Verification items for the finished model (mm, model axes). Give positions to 0.01 mm unless a question says otherwise; leave off trailing zeros. Write each loop counter-clockwise with the first axis right and the second up, starting at its lowest first coordinate (ties: lowest second). Pieces come first, ordered by that corner, then holes. Notation, with made-up numbers: (76, 37) -> (103, 37) arc R27 ccw to (103, 67) -> close; hole circle Ø9 at (66, 43). An arc over 180 degrees is marked (long way). Answer as CSV lines item,"result". Start each with the question number.
1) Material ranges on L1, parallel to X at y = 19, z = 0.5; L2, parallel to Z at x = 0, y = -43, recorded low to high.
2) Sectioned sample at A-A on z = 0. Record the cut outline in (x, y), and give its area (3 significant figures).
3) Sectioned sample at B-B on z = -15. Record the cut outline in (x, y), and give its area (3 significant figures).
4) Gauge pin test, flat ends, axial feed: pin 1 Ø10 at (x, y) = (8, -25) entering from -Z; pin 2 Ø12 at (x, y) = (15.5, -35) entering from +Z; pin 3 Ø10.5 at (x, z) = (1, -5) entering from +Y; pin 4 Ø1.5 at (y, z) = (21.5, -7) entering from -X. Record the tip position at first contact, or that the pin passes through.
5) Sectioned sample at C-C on y = -7. Record the cut outline in (x, z) (1 decimal), and give its area (3 significant figures).
6) Sectioned sample at D-D on x = 16.5. Record the cut outline in (y, z).
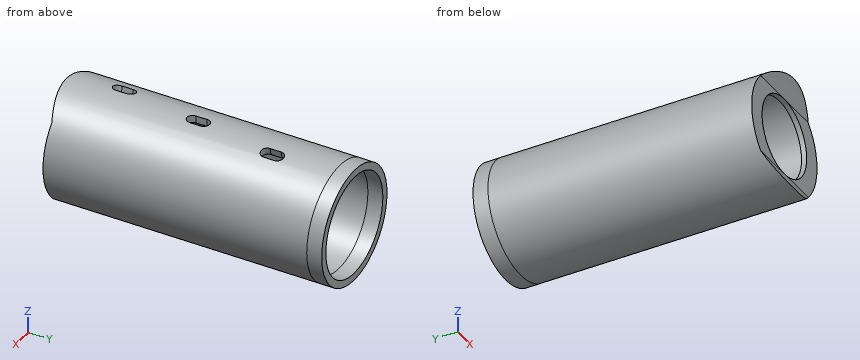
```python
from build123d import *

# Parameters (mm, degrees)
F0_R          = 20.0025
F0_R_2        = 17.4625
F1_DEPTH      = 47.5
F2_R          = 20.0025
F2_R_2        = 13.6525
F3_DEPTH      = 5.08
F5_DEPTH      = 20.0035
F5_DEPTH_BACK = 20.0035
F7_DEPTH      = 20.0035001
F11_DEPTH     = 23.7251510989
F14_DEPTH     = 23.7251510989
F15_R         = 20.0025
F15_R_2       = 17.4625
F16_DEPTH     = 5.207


with BuildPart() as f1:
    # F0 (on Front) → F1 (new body, symmetric)
    with BuildSketch(Plane.XZ):
        Circle(F0_R)
        Circle(F0_R_2, mode=Mode.SUBTRACT)
    extrude(amount=F1_DEPTH, both=True)

    # F2 (on face) → F3 (join)
    with BuildSketch(Plane.XZ.offset(47.5)):
        Circle(F2_R)
        Circle(F2_R_2, mode=Mode.SUBTRACT)
    extrude(amount=-F3_DEPTH)

    # F4 (on Right) → F5 (cut, two sides)
    with BuildSketch(Plane.YZ) as f5_sk:
        with BuildLine():
            Line((-44.198, -13.6525), (-44.198, 13.6525))
            ThreePointArc((-44.198, 13.6525), (-45.6936183213, 16.9082984729), (-47.5, 20.0025))
            Line((-47.5, 20.0025), (-47.5, -20.0025))
            ThreePointArc((-47.5, -20.0025), (-45.6936183213, -16.9082984729), (-44.198, -13.6525))
        make_face()
    extrude(amount=-F5_DEPTH, mode=Mode.SUBTRACT)
    extrude(f5_sk.sketch, amount=F5_DEPTH_BACK, mode=Mode.SUBTRACT)

    # F6 (on Top) → F7 (cut, through all)
    with BuildSketch(Plane.XY):
        with BuildLine():
            Line((-2.032, 0.379), (-2.032, -3.431))
            ThreePointArc((-2.032, -3.431), (0, -5.463), (2.032, -3.431))
            Line((2.032, -3.431), (2.032, 0.379))
            ThreePointArc((2.032, 0.379), (0, 2.411), (-2.032, 0.379))
        make_face()
    extrude(amount=F7_DEPTH, mode=Mode.SUBTRACT)

    # F10 (on face) → F11 (cut, through all)
    with BuildSketch(Plane(origin=(0, 0, 0), x_dir=(0.9781476007, 0, 0.2079116908), z_dir=(0.2079116908, 0, -0.9781476007))):
        with BuildLine():
            ThreePointArc((2.032, 31.498), (0, 33.53), (-2.032, 31.498))
            Line((-2.032, 31.498), (-2.032, 27.688))
            ThreePointArc((-2.032, 27.688), (0, 25.656), (2.032, 27.688))
            Line((2.032, 27.688), (2.032, 31.498))
        make_face()
    extrude(amount=-F11_DEPTH, mode=Mode.SUBTRACT)

    # F13 (on face) → F14 (cut, through all)
    with BuildSketch(Plane(origin=(0, 0, 0), x_dir=(0.9781476007, 0, -0.2079116908), z_dir=(-0.2079116908, 0, -0.9781476007))):
        with BuildLine():
            Line((2.032, -28.446), (2.032, -24.636))
            ThreePointArc((2.032, -24.636), (0, -22.604), (-2.032, -24.636))
            Line((-2.032, -24.636), (-2.032, -28.446))
            ThreePointArc((-2.032, -28.446), (0, -30.478), (2.032, -28.446))
        make_face()
    extrude(amount=-F14_DEPTH, mode=Mode.SUBTRACT)

    # F15 (on face) → F16 (join)
    with BuildSketch(Plane(origin=(0, 47.5, 0), x_dir=(-1, 0, 0), z_dir=(0, 1, 0))):
        Circle(F15_R)
        Circle(F15_R_2, mode=Mode.SUBTRACT)
    extrude(amount=F16_DEPTH)


solid = f1.part
```
Ans:
1,L1,"x = -20 to -17.46, 17.46 to 20"
1,L2,"z = -20 to -13.65, 13.65 to 20"
2,outline,"(-20, -44.2) -> (-13.65, -44.2) -> (-13.65, -42.42) -> (-17.46, -42.42) -> (-17.46, 52.71) -> (-20, 52.71) -> close; (13.65, -44.2) -> (20, -44.2) -> (20, 52.71) -> (17.46, 52.71) -> (17.46, -42.42) -> (13.65, -42.42) -> close"
2,area,"506 mm²"
3,outline,"(-13.23, -44.77) -> (13.23, -44.77) -> (13.23, 52.71) -> (8.94, 52.71) -> (8.94, -42.42) -> (-8.94, -42.42) -> (-8.94, 52.71) -> (-13.23, 52.71) -> close"
3,area,"879 mm²"
4,pin 1,"stops at z = -19.78"
4,pin 2,"stops at z = 17.6"
4,pin 3,"passes through"
4,pin 4,"stops at x = -19"
5,outline,"circle Ø40 at (0, 0); hole circle Ø34.9 at (0, 0)"
5,area,"299 mm²"
6,outline,"(-44.2, -11.31) -> (52.71, -11.31) -> (52.71, -5.72) -> (-42.42, -5.72) -> (-42.42, 5.72) -> (52.71, 5.72) -> (52.71, 11.31) -> (-44.2, 11.31) -> close"
